The model under review builds one solid part; all positions refer to its coordinate system, in mm. Face numbers are marked on the shaded views. Coordinates: 2 decimals unless noted, no trailing zeros. Loops run counter-clockwise (first coordinate to the right, second up) from the corner with the lowest first, then second, coordinate; pieces in that order, holes last. Notation, with made-up numbers: M 59.25,86.25 L 73.25,86.25 A6 cw 73.25,94.25 Z; hole C 83.25,62 d3. An arc over 180 degrees is marked long. Use CSV: the item, a comma, the result in double quotes. Start each with the question number.
1. Add section C-C, the plane z = 7. State how many separate pieces and enclosed holes the cut face has, then the cut area to 3 significant figures.
2. Add section A-A, the plane x = 66. Write out the cut boundary in (y, z).
3. Add section B-B, the plane y = -2.5. Write out the cut boundary in (x, z).
4. Add section D-D, the plane y = -29. Write out the cut boundary in (x, z).
5. Clearance check with flat-ended pins moving along their axes: P1, Ø2, axis at x = 35.5, z = 2, coming from the -Y side; P2, Ø3.5, axis at x = 60, y = -29, coming from the +Z side; P3, Ø1.9, axis at x = 14, y = -16, coming from the +Z side; P4, Ø1.4, axis at x = 54.5, y = 33, coming from the -Z side. State where each tip first meets the part, or that it passes through.
6. Draft analysis for pull direction Y (two halves, no side actions). For the marked faces 1 and 2, state which applies: +Y half, -Y half, draft (parallel to the pull), parting line (faces both ways), or undercut.
7. For L1, parallel to Y at x = 7, z = 3.75 (3 decimals); L2, parallel to Y at x = 57, z = 5.25; L3, parallel to Y at x = 57, z = 6.55, list the stretches that pass through material, from the lowest coordinate up.
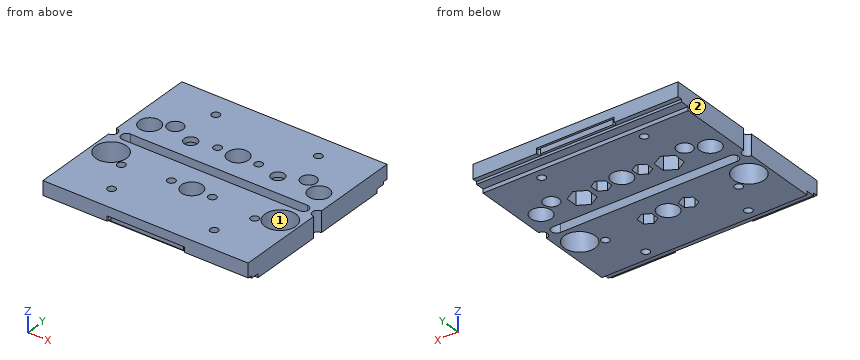
from build123d import *

# Parameters (mm, degrees)
SKETCH_2_W           = 80
SKETCH_2_H           = 34
SKETCH_2_R           = 4.05
EXTRUDE_1_DEPTH      = 8
SKETCH_3_R           = 2.55
CUT_EXTRUDE_1_DEPTH  = 88.292611371
CUT_EXTRUDE_2_DEPTH  = 88.292611371
SKETCH_5_R           = 1.55
CUT_EXTRUDE_3_DEPTH  = 88.292611371
CUT_EXTRUDE_5_DEPTH  = 4.5
SKETCH_25_R          = 1.55
CUT_EXTRUDE_13_DEPTH = 88.292611371
CUT_EXTRUDE_11_DEPTH = 2
EXTRUDE_2_DEPTH      = 8
SKETCH_26_R          = 6.025
CUT_EXTRUDE_14_DEPTH = 89.926936302
SKETCH_27_R          = 3
SKETCH_27_R_2        = 1.55
CUT_EXTRUDE_15_DEPTH = 89.926936302
CUT_EXTRUDE_16_DEPTH = 6


with BuildPart() as part:
    # Sketch 2 → Extrude 1 (new body)
    with BuildSketch(Plane.XY):
        with Locations((40, 17)):
            Rectangle(SKETCH_2_W, SKETCH_2_H)
        with Locations((7, 8)):
            Circle(SKETCH_2_R, mode=Mode.SUBTRACT)
        with Locations((40, 10)):
            Circle(SKETCH_2_R, mode=Mode.SUBTRACT)
        with Locations((73, 8)):
            Circle(SKETCH_2_R, mode=Mode.SUBTRACT)
    extrude_1 = extrude(amount=EXTRUDE_1_DEPTH)

    # Sketch 3 → Cut-Extrude 1 (cut, through all)
    with BuildSketch(Plane.XY.offset(8)):
        with Locations((23, 8)):
            Circle(SKETCH_3_R)
        with Locations((57, 8)):
            Circle(SKETCH_3_R)
    extrude(amount=-CUT_EXTRUDE_1_DEPTH, mode=Mode.SUBTRACT)

    # Sketch 4 → Cut-Extrude 2 (cut, through all)
    with BuildSketch(Plane(origin=(80, 0, 0), x_dir=(0, 0, -1), z_dir=(1, 0, 0))):
        Polygon((-1.5, 32.2), (-2.5, 32.2), (-2.5, 34), (0, 34), (0, 28.8), (-1.5, 28.8), align=None)
    cut_extrude_2 = extrude(amount=-CUT_EXTRUDE_2_DEPTH, mode=Mode.SUBTRACT)

    # Sketch 5 → Cut-Extrude 3 (cut, through all)
    with BuildSketch(Plane.XY.offset(8)):
        with Locations((48, 10)):
            Circle(SKETCH_5_R)
        with Locations((32, 10)):
            Circle(SKETCH_5_R)
    cut_extrude_3 = extrude(amount=-CUT_EXTRUDE_3_DEPTH, mode=Mode.SUBTRACT)

    # Sketch 8 → Cut-Extrude 5 (cut)
    with BuildSketch(Plane(origin=(0, 0, 0), x_dir=(-1, 0, 0), z_dir=(0, 0, -1))):
        Polygon((-45.15, 8.354551733), (-45.15, 11.645448267), (-48, 13.290896534), (-50.85, 11.645448267), (-50.85, 8.354551733), (-48, 6.709103466), align=None)
        Polygon((-29.15, 8.354551733), (-29.15, 11.645448267), (-32, 13.290896534), (-34.85, 11.645448267), (-34.85, 8.354551733), (-32, 6.709103466), align=None)
    cut_extrude_5 = extrude(amount=-CUT_EXTRUDE_5_DEPTH, mode=Mode.SUBTRACT)

    # Sketch 25 → Cut-Extrude 13 (cut, through all)
    with BuildSketch(Plane(origin=(0, 0, 0), x_dir=(-1, 0, 0), z_dir=(0, 0, -1))):
        with Locations((-60, 25)):
            Circle(SKETCH_25_R)
        with Locations((-20, 25)):
            Circle(SKETCH_25_R)
    cut_extrude_13 = extrude(amount=-CUT_EXTRUDE_13_DEPTH, mode=Mode.SUBTRACT)

    # Sketch 19 → Cut-Extrude 11 (cut)
    with BuildSketch(Plane(origin=(0, 0, 2.5), x_dir=(-1, 0, 0), z_dir=(0, 0, -1))):
        with BuildLine():
            Line((-25, 34), (-55.247938178, 34))
            Line((-55.247938178, 34), (-55.247938178, 33.2))
            ThreePointArc((-55.247938178, 33.2), (-54.747938178, 32.7), (-54.247938178, 33.2))
            Line((-54.247938178, 33.2), (-26, 33.2))
            ThreePointArc((-26, 33.2), (-25.5, 32.7), (-25, 33.2))
            Line((-25, 33.2), (-25, 34))
        make_face()
    cut_extrude_11 = extrude(amount=-CUT_EXTRUDE_11_DEPTH, mode=Mode.SUBTRACT)

    # Sketch 22 → Extrude 2 (add)
    with BuildSketch(Plane.XY.offset(8)):
        with BuildLine():
            Line((0, -4), (5.5, -4))
            ThreePointArc((5.5, -4), (3.5, -2), (5.5, 0))
            Line((5.5, 0), (0, 0))
            ThreePointArc((0, 0), (2, -2), (0, -4))
        make_face()
        with BuildLine():
            Line((80, 0), (74.5, 0))
            ThreePointArc((74.5, 0), (76.5, -2), (74.5, -4))
            Line((74.5, -4), (80, -4))
            ThreePointArc((80, -4), (78, -2), (80, 0))
        make_face()
    extrude(amount=-EXTRUDE_2_DEPTH)

    # Mirror 2: Extrude 1, Cut-Extrude 2, Cut-Extrude 3, Cut-Extrude 5, Cut-Extrude 13, Cut-Extrude 11 across plane
    add(extrude_1.mirror(Plane(origin=(0, -2, 0), x_dir=(0, 0, 1), z_dir=(0, -1, 0))))
    add(cut_extrude_2.mirror(Plane(origin=(0, -2, 0), x_dir=(0, 0, 1), z_dir=(0, -1, 0))), mode=Mode.SUBTRACT)
    add(cut_extrude_3.mirror(Plane(origin=(0, -2, 0), x_dir=(0, 0, 1), z_dir=(0, -1, 0))), mode=Mode.SUBTRACT)
    add(cut_extrude_5.mirror(Plane(origin=(0, -2, 0), x_dir=(0, 0, 1), z_dir=(0, -1, 0))), mode=Mode.SUBTRACT)
    add(cut_extrude_13.mirror(Plane(origin=(0, -2, 0), x_dir=(0, 0, 1), z_dir=(0, -1, 0))), mode=Mode.SUBTRACT)
    add(cut_extrude_11.mirror(Plane(origin=(0, -2, 0), x_dir=(0, 0, 1), z_dir=(0, -1, 0))), mode=Mode.SUBTRACT)

    # Sketch 26 → Cut-Extrude 14 (cut, through all)
    with BuildSketch(Plane(origin=(0, 0, 0), x_dir=(-1, 0, 0), z_dir=(0, 0, -1))):
        with Locations((-73, -12)):
            Circle(SKETCH_26_R)
        with Locations((-7, -12)):
            Circle(SKETCH_26_R)
    extrude(amount=-CUT_EXTRUDE_14_DEPTH, mode=Mode.SUBTRACT)

    # Sketch 27 → Cut-Extrude 15 (cut, through all)
    with BuildSketch(Plane(origin=(0, 0, 0), x_dir=(-1, 0, 0), z_dir=(0, 0, -1))):
        with Locations((-66, 12)):
            Circle(SKETCH_27_R)
        with Locations((-66, -16)):
            Circle(SKETCH_27_R_2)
        with Locations(Location((-14, -16, 0), (0, 0, 180))):
            Circle(SKETCH_27_R_2)
        with Locations(Location((-14, 12, 0), (0, 0, 180))):
            Circle(SKETCH_27_R)
    extrude(amount=-CUT_EXTRUDE_15_DEPTH, mode=Mode.SUBTRACT)

    # Sketch 28 → Cut-Extrude 16 (cut)
    with BuildSketch(Plane(origin=(0, 0, 0), x_dir=(-1, 0, 0), z_dir=(0, 0, -1))):
        Polygon((-52.9, 5.632863896), (-52.9, 10.367136104), (-57, 12.734272207), (-61.1, 10.367136104), (-61.1, 5.632863896), (-57, 3.265727793), align=None)
        Polygon((-18.9, 5.632863896), (-18.9, 10.367136104), (-23, 12.734272207), (-27.1, 10.367136104), (-27.1, 5.632863896), (-23, 3.265727793), align=None)
    extrude(amount=-CUT_EXTRUDE_16_DEPTH, mode=Mode.SUBTRACT)


solid = part.part
Computed:
1,separate pieces,"1"
1,enclosed holes,"21"
1,area,"4,850 mm^2"
2,outline,"M -38,2.5 L -36.2,2.5 L -36.2,1.5 L -32.8,1.5 L -32.8,0 L -17.55,0 L -17.55,8 L -38,8 Z; M -14.45,0 L -4,0 L -4,8 L -14.45,8 Z; M 0,0 L 9,0 L 9,8 L 0,8 Z; M 15,0 L 28.8,0 L 28.8,1.5 L 32.2,1.5 L 32.2,2.5 L 34,2.5 L 34,8 L 15,8 Z"
3,outline,"M 1.94,0 L 3.56,0 L 3.56,8 L 1.94,8 Z; M 76.44,0 L 78.06,0 L 78.06,8 L 76.44,8 Z"
4,outline,"M 0,0 L 18.45,0 L 18.45,8 L 0,8 Z; M 21.55,0 L 58.45,0 L 58.45,8 L 21.55,8 Z; M 61.55,0 L 80,0 L 80,8 L 61.55,8 Z"
5,P1,"stops at y = -37.2"
5,P2,"stops at z = 8"
5,P3,"passes through"
5,P4,"stops at z = 2.5"
6,face 1,"undercut"
6,face 2,"draft"
7,L1,"y = -38 to -18.025, -5.975 to -4, 0 to 3.95, 12.05 to 34"
7,L2,"y = -38 to -4, 0 to 3.27, 12.73 to 34"
7,L3,"y = -38 to -4, 0 to 5.45, 10.55 to 34"
